Work out the finished part from the listing and answer in its coordinate system (mm). A direction names the side the tool comes from. Coordinates: 2 decimals unless noted, no trailing zeros. Order: outer loops, then holes, each group sorted by start corner. A loop starts at its lowest first (then second) coordinate and runs counter-clockwise, first axis right, second up. Notation, with made-up numbers: M 44.5,71.5 L 54.5,71.5 A23 ccw 54.5,105.5 Z; hole C 52,-26 d3. An arc over 180 degrees is marked long. Use a Markdown table: item, result. Add a question column.
Autodesk Inventor part; units mm, degrees
ref_plane "YZ Plane" through (0, 0, 0) normal (1, 0, 0) x (0, 1, 0)
ref_plane "XZ Plane" through (0, 0, 0) normal (0, 1, 0) x (-1, 0, 0)
ref_plane "XY Plane" through (0, 0, 0) normal (0, 0, 1) x (1, 0, 0)
sketch "Skizze1" plane through (0, 0, 0) normal (0, 1, 0) x (-1, 0, 0)
  line L0 (-5, 7) -> (5, 7)
  line L1 (5, 7) -> (5, -7)
  line L2 (5, -7) -> (-5, -7)
  line L3 (-5, -7) -> (-5, 7)
  line L4 (-5, 7) -> (5, -7) construction
  line L5 (5, 7) -> (-5, -7) construction
  line L6 (5, 4.5) -> (-1.5, 4.5)
  line L7 (-1.5, 4.5) -> (-1.5, -4.5)
  line L8 (-1.5, -4.5) -> (5, -4.5)
  line L9 (5, -4.5) -> (5, 4.5)
  line L10 (5, 4.5) -> (-1.5, -4.5) construction
  line L11 (-1.5, 4.5) -> (5, -4.5) construction
  line L12 (7, 0) -> (-7, 0)
  point P0 (0, 0)
  point P1 (1.75, 0)
  point P2 (1.75, 0)
  dimension "d0" = 10
  dimension "d1" = 14
  dimension "d2" = 6.5
  dimension "d3" = 9
extrude "Extrusion1" add sketch "Skizze1" along normal blind 30 contours L0 L1 L6 L7 L12 L3 | L12 L7 L8 L1 L2 L3
sketch "Skizze2" plane through (5, 0, 7) normal (1, 0, 0) x (0, 0, -1)
  line L0 (7, -6) -> (7, 36) construction
  point P0 (7, 0)
  point P1 (7, 25)
  point P2 (7, 5)
  dimension "d6" = 20
  dimension "d7" = 5
hole "Bohrung1" at (5, 25, 0) at (5, 5, 0) direction (-1, 0, 0) diameter 5 end through all counterbore diameter 8 counterbore depth 2
sketch "Skizze3" plane through (0, 30, 0) normal (0, 1, 0) x (1, 0, 0)
  line L0 (-5, 4.5) -> (1.5, 4.5)
  line L1 (1.5, 4.5) -> (1.5, -4.5)
  line L2 (1.5, -4.5) -> (-5, -4.5)
  line L3 (-5, -4.5) -> (-5, -7)
  line L4 (-5, -7) -> (5, -7)
  line L5 (5, -7) -> (5, 7)
  line L6 (5, 7) -> (-5, 7)
  line L7 (-5, 7) -> (-5, 4.5)
  line L8 (5, 7) -> (-5, 7)
  line L9 (-5, -7) -> (-5, -20)
  line L10 (-5, -20) -> (19, -20)
  line L11 (19, -20) -> (19, -16)
  line L12 (19, -16) -> (5, -16)
  line L13 (5, -7) -> (5, 7)
  line L14 (5, -16) -> (5, -7)
  point P0 (0, 0)
  dimension "d16" = 20
  dimension "d17" = 14
  dimension "d18" = 4
extrude "Extrusion2" add sketch "Skizze3" against normal blind 30 and the other way blind 15 contours L14 L12 L11 L10 L9 L4
sketch "Skizze4" plane through (19, 0, 16) normal (0, 0, -1) x (-1, 0, 0)
  line L0 (0, 0) -> (0, 45)
  line L1 (14, 0) -> (0, 0)
  line L2 (14, 0) -> (14, 45)
  line L3 (0, 45) -> (14, 45)
  line L4 (24, 45) -> (0, 45)
  line L5 (7, 45) -> (7, 0) construction
  line L6 (14, 0) -> (0, 0)
  line L7 (7, 40) -> (7, 5) construction
  line L8 (5.25, 40) -> (5.25, 5)
  line L9 (8.75, 5) -> (8.75, 40)
  arc A0 (8.75, 40) -> (5.25, 40) centre (7, 40) ccw
  arc A1 (5.25, 5) -> (8.75, 5) centre (7, 5) ccw
  point P0 (19, 0)
  point P1 (7, 22.5)
  dimension "d23" = 3.5
  dimension "d24" = 5
  dimension "d25" = 5
extrude "Extrusion3" cut sketch "Skizze4" against normal blind 30 contours A0 L9 A1 L8
properties part number "Schlitten_Part2"
(1) Given P1, Ø6.5, axis at y = 24, z = -0.5, coming from the +X side; P2, Ø3, axis at x = 1, y = 40, coming from the -Z side; P3, Ø8, axis at x = 2, z = 2.5, coming from the +Y side; P4, Ø4.5, axis at y = 25, z = 0, coming from the -X side, each flat-ended and moving along its own axis, determine where each tip first touches the part or whether it passes through.
(2) A cutting plane is placed at D-D on y = 14. Write down the section's boundary in (x, z).
(3) The mould has two halves that part along X. Classify faces 1 (the flat face through (1.5, 15, 0)), 2 (the cylindrical face through (12.04, 3.25, 17.97)), 3 (the flat face through (0, 38, 7)): pulls with the +X half, pulls with the -X half, needs draft (parallel to the pull), parting line crosses it, or undercut.
(4) A cutting plane is placed at A-A on y = 25. Write down the section's boundary in (x, z), plus the area to 3 significant figures.
(5) A cutting plane is placed at B-B on x = 1. Write down the section's boundary in (y, z).
(6) Which of the six approach directions +Z, -Z, +X, -X, +Y, -Y give full straight-line access (tool end or side, diameter ignored) to faces 4 (the flat face through (13.75, 23, 18)), 5 (the flat face through (2, 30, 0)), 6 (the flat face through (-2, 15, -4.5)), 7 (the cylindrical face through (3.986, 21.034, 0.521)), 8 (the flat face through (5, 17, 7))?
(7) Straight lines are drawn through the part: line 1 (Y direction, x = 4, z = 0); line 2 (Y direction, x = 2.35, z = 0); line 3 (Z direction, x = 2.3, y = 5). For each, find the intervals that lie inside material, in ascending order.
(8) A cutting plane is placed at C-C on z = 18.75. Write down the section's boundary in (x, y), plus the area to 3 significant figures.
From the geometry:
| question | item | result |
|---|---|---|
| 1 | P1 | stops at x = 5 |
| 1 | P2 | stops at z = 7 |
| 1 | P3 | stops at y = 30 |
| 1 | P4 | passes through |
| 2 | outline | M -5,-7 L 5,-7 L 5,16 L 10.25,16 L 10.25,20 L -5,20 L -5,4.5 L 1.5,4.5 L 1.5,-4.5 L -5,-4.5 Z; M 13.75,16 L 19,16 L 19,20 L 13.75,20 Z |
| 3 | face 1 | pulls with the -X half |
| 3 | face 2 | undercut |
| 3 | face 3 | needs draft |
| 4 | outline | M -5,-7 L 5,-7 L 5,-4 L 3,-4 L 3,-2.5 L 1.5,-2.5 L 1.5,-4.5 L -5,-4.5 Z; M -5,4.5 L 1.5,4.5 L 1.5,2.5 L 3,2.5 L 3,4 L 5,4 L 5,16 L 10.25,16 L 10.25,20 L -5,20 Z; M 13.75,16 L 19,16 L 19,20 L 13.75,20 Z |
| 4 | area | 230 mm2 |
| 5 | outline | M 0,-7 L 30,-7 L 30,-4.5 L 0,-4.5 Z; M 0,4.5 L 30,4.5 L 30,7 L 45,7 L 45,20 L 0,20 Z |
| 6 | face 4 | +Z, -Z |
| 6 | face 5 | -Z, +X, -X, +Y |
| 6 | face 6 | -X, +Y, -Y |
| 6 | face 7 | +X |
| 6 | face 8 | -Z, +X, +Y, -Y |
| 7 | line 1 | y = 0 to 1, 9 to 21, 29 to 30 |
| 7 | line 2 | y = 0 to 2.5, 7.5 to 22.5, 27.5 to 30 |
| 7 | line 3 | z = -7 to -2.5, 2.5 to 20 |
| 8 | outline | M -5,0 L 19,0 L 19,45 L -5,45 Z; hole M 10.25,5 A1.75 ccw 13.75,5 L 13.75,40 A1.75 ccw 10.25,40 Z |
| 8 | area | 948 mm2 |
